Part print with two shaded views. Sizes in mm from the minimum x, y, z corner. A direction names the side the tool comes from. Coordinates: 2 decimals unless noted, no trailing zeros. Loops run counter-clockwise (first coordinate to the right, second up) from the corner with the lowest first, then second, coordinate; pieces in that order, holes last. Notation, with made-up numbers: (71, 48.25) -> (129, 48.25) arc R11 cw to (129, 65.25) -> close; hole circle Ø10 at (64, 43.25). An arc over 180 degrees is marked (long way). Use one line per item in the form item = value.
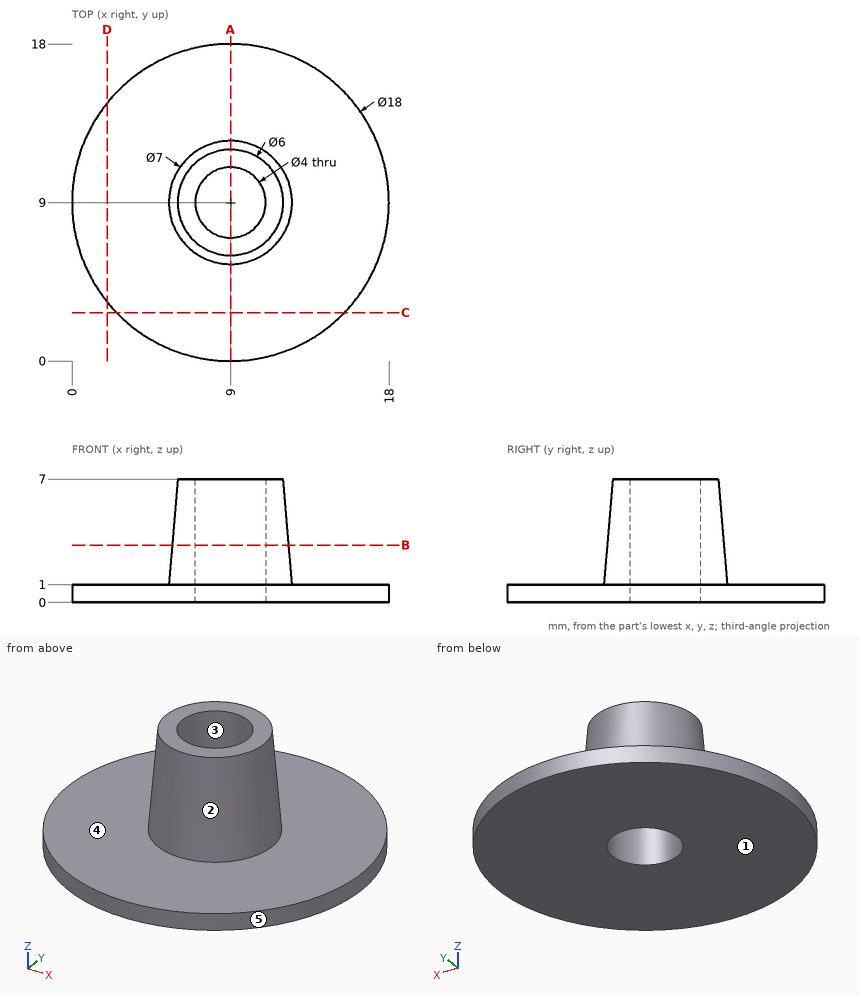
Q1. Band-saw the part on A-A, the plane x = 9. Write the cut outline in (y, z), and give its area (3 significant figures).
Result:
outline = (0, 0) -> (7, 0) -> (7, 7) -> (6, 7) -> (5.5, 1) -> (0, 1) -> close; (11, 0) -> (18, 0) -> (18, 1) -> (12.5, 1) -> (12, 7) -> (11, 7) -> close
area = 29.0 mm2
Q2. Which spindle directions (+Z, -Z, +X, -X, +Y, -Y) get a long thin tool onto all of the face, cutting with end or side? Do the marked faces 4 and 5. Say none if no direction does.
Result:
face_4 = +Z
face_5 = +Z, -Z
Q3. Band-saw the part on D-D, the plane x = 2. Write the cut outline in (y, z).
Result:
outline = (3.34, 0) -> (14.66, 0) -> (14.66, 1) -> (3.34, 1) -> close
Q4. Mould opens along X. For the marked faces 1, 2 and 3 say: released by +X, released by -X, zero draft, split by the parting line, or undercut.
Result:
face_1 = zero draft
face_2 = split by the parting line
face_3 = undercut
Q5. Pin check, flat tips, straight feed: pin 1 Ø2 at (x, y) = (12, 3.5) entering from +Z; pin 2 Ø10 at (x, y) = (3.5, 11.5) entering from +Z; pin 3 Ø3 at (y, z) = (15, 1.5) entering from +X; pin 4 Ø3 at (x, z) = (4.5, 3.5) entering from -Y. Stop position of each tip, or through.
Result:
pin_1 = 1
pin_2 = 7
pin_3 = 16.74
pin_4 = 7.63
Q6. Wall check: line 1 along Z through (x, y) = (1.75, 8.5); line 2 along Y through (x, z) = (9, 1.5); line 3 along Y through (x, z) = (9, 4.75). Give the ranges that are in metal, low to high.
Result:
line_1 = 0 to 1
line_2 = 5.54 to 7, 11 to 12.46
line_3 = 5.81 to 7, 11 to 12.19
Q7. Band-saw the part on C-C, the plane y = 2.75. Write the cut outline in (x, z).
Result:
outline = (2.52, 0) -> (15.48, 0) -> (15.48, 1) -> (2.52, 1) -> close
Q8. Band-saw the part on B-B, the plane z = 3.25. Write the cut outline in (x, y) (1 decimal), and give its area (3 significant figures).
Result:
outline = circle Ø6.6 at (9, 9); hole circle Ø4 at (9, 9)
area = 21.9 mm2
